Drawing for the job (mm, zero at the part's lowest x, y, z). Round coordinates to 2 decimals unless told otherwise and drop trailing zeros. Write each loop counter-clockwise with the first axis right and the second up, starting at its lowest first coordinate (ties: lowest second). Pieces come first, ordered by that corner, then holes.
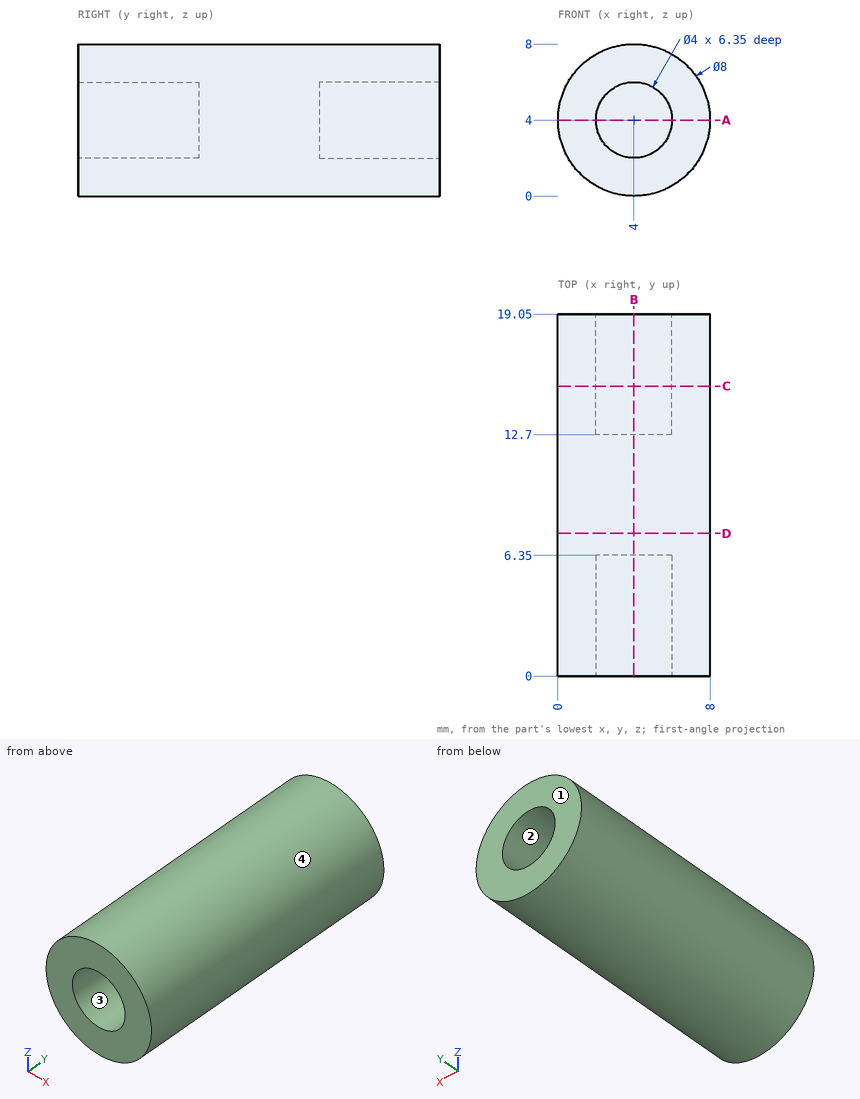
Q1. Saw through at C-C, the plane y = 15.25. Write the cut outline in (x, z), and give its area (3 significant figures).
Q2. Two-plate mould, pull along Z, no slides. Class the marked faces 1, 2, 3 and 4: released by +Z, released by -Z, zero draft, split by the parting line, or undercut.
Q3. Drop flat-ended pins along their axis: P1, Ø3, axis at y = 15, z = 1.5, coming from the +X side; P2, Ø2.5, axis at x = 4, z = 4, coming from the +Y side; P3, Ø3.5, axis at x = 4, z = 4, coming from the -Y side. Give the stop position or say it passes through.
Q4. Saw through at D-D, the plane y = 7.5. Write the cut outline in (x, z), and give its area (3 significant figures).
Q5. Saw through at B-B, the plane x = 4. Write the cut outline in (y, z).
Q6. Saw through at A-A, the plane z = 4. Write the cut outline in (x, y).
Q7. Wall check: line 1 (X direction, y = 15.75, z = 4); line 2 (Y direction, x = 2.5, z = 4.5); line 3 (X direction, y = 16.75, z = 4.5). Give the ranges that are in metal, low to high.
Computed:
1. outline: circle Ø8 at (4, 4); hole circle Ø4 at (4, 4)
1. area: 37.7 mm2
2. face 1: zero draft
2. face 2: undercut
2. face 3: undercut
2. face 4: split by the parting line
3. P1: stops at x = 7.87
3. P2: stops at y = 12.7
3. P3: stops at y = 6.35
4. outline: circle Ø8 at (4, 4)
4. area: 50.3 mm2
5. outline: (0, 0) - (19.05, 0) - (19.05, 2) - (12.7, 2) - (12.7, 6) - (19.05, 6) - (19.05, 8) - (0, 8) - (0, 6) - (6.35, 6) - (6.35, 2) - (0, 2) - close
6. outline: (0, 0) - (2, 0) - (2, 6.35) - (6, 6.35) - (6, 0) - (8, 0) - (8, 19.05) - (6, 19.05) - (6, 12.7) - (2, 12.7) - (2, 19.05) - (0, 19.05) - close
7. line 1: x = 0 to 2, 6 to 8
7. line 2: y = 6.35 to 12.7
7. line 3: x = 0.03 to 2.06, 5.94 to 7.97
